Could you check a few things on this drawing? It's one solid part, dimensions in mm from its lowest x, y, z. A direction names the side the tool comes from. Round coordinates to 2 decimals unless told otherwise and drop trailing zeros. Loops run counter-clockwise (first coordinate to the right, second up) from the corner with the lowest first, then second, coordinate; pieces in that order, holes last. Notation, with made-up numbers: M 37,72.5 L 70,72.5 A22 ccw 70,108.5 Z; hole C 39.5,72 d9. An arc over 180 degrees is marked long. Put each result on its own line as item: value. Start each with the question number.
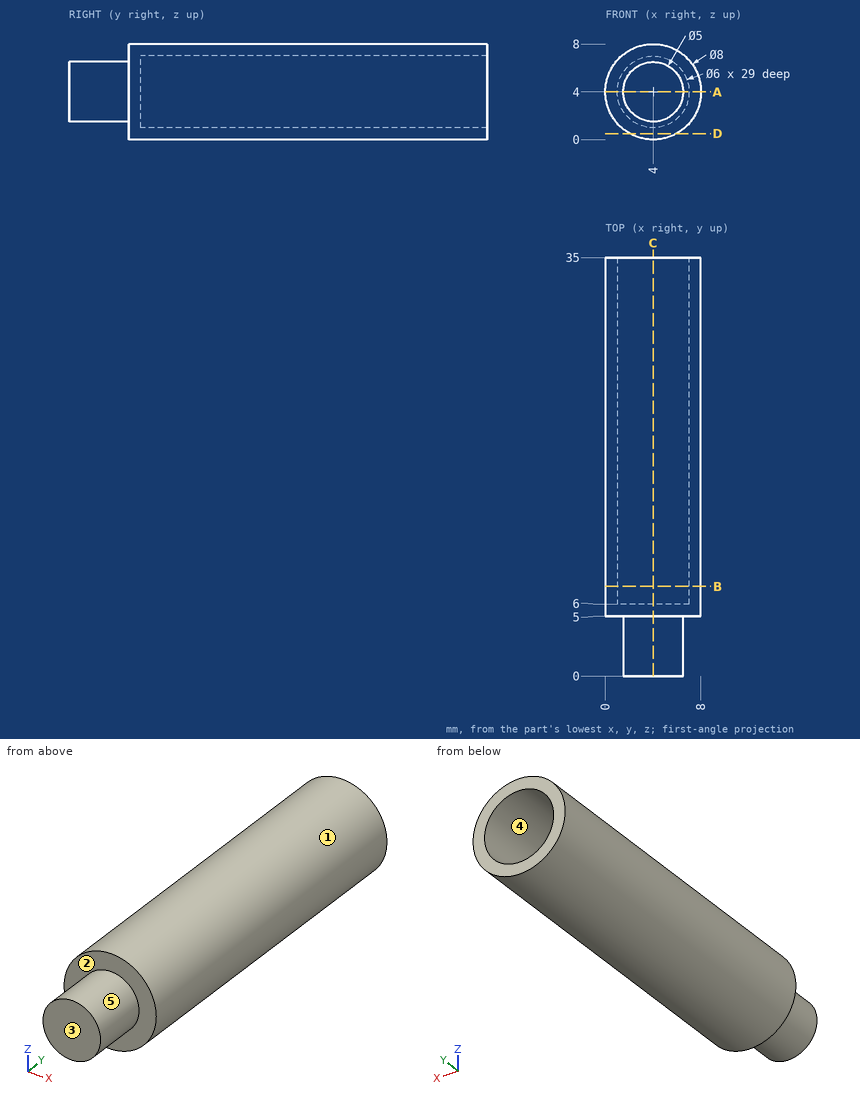
1) Suppose I cut it at D-D (z = 0.5). Write out the boundary of the cut face in (x, y), plus the area to 3 significant figures.
2) I'm going to push a flat-ended pin straight in: P1, Ø3, axis at x = 3.5, z = 5, coming from the +Y side. Where does the tip first touch, or does it pass through?
3) Suppose I cut it at C-C (x = 4). Write out the boundary of the cut face in (y, z), plus the area to 3 significant figures.
4) On a 3-axis mill with a long thin cutter (end or side, diameter ignored), from which of +Z, -Z, +X, -X, +Y, -Y can I reach the whole of each face in a straight line? I mean the marked faces 1 and 2. Say none if no direction works.
5) Suppose I cut it at A-A (z = 4). Write out the boundary of the cut face in (x, y).
6) If I drill on probe 1 along Z at (x, y) = (4, 12); probe 2 along Y at (x, z) = (6.5, 3.25), over which ranges is the centre line in solid material (lowest first)? Write a range as from..to.
7) Suppose I cut it at B-B (y = 7.5). Write out the boundary of the cut face in (x, z), plus the area to 3 significant figures.
8) If we mould it in two halves opening along Z, with no side actions, what happens to the marked faces 3, 4 and 5? For each: pulls with the +Z half, pulls with the -Z half, needs draft (parallel to the pull), parting line crosses it, or undercut.
Results are:
1. outline: M 2.06,5 L 5.94,5 L 5.94,35 L 2.06,35 Z
1. area: 116 mm²
2. P1: y = 6
3. outline: M 0,1.5 L 5,1.5 L 5,0 L 35,0 L 35,1 L 6,1 L 6,7 L 35,7 L 35,8 L 5,8 L 5,6.5 L 0,6.5 Z
3. area: 91.0 mm²
4. face 1: +Y, -Y
4. face 2: -Y
5. outline: M 0,5 L 1.5,5 L 1.5,0 L 6.5,0 L 6.5,5 L 8,5 L 8,35 L 7,35 L 7,6 L 1,6 L 1,35 L 0,35 Z
6. probe 1: 0..1, 7..8
6. probe 2: 5..6
7. outline: C 4,4 d8; hole C 4,4 d6
7. area: 22.0 mm²
8. face 3: needs draft
8. face 4: undercut
8. face 5: parting line crosses it
